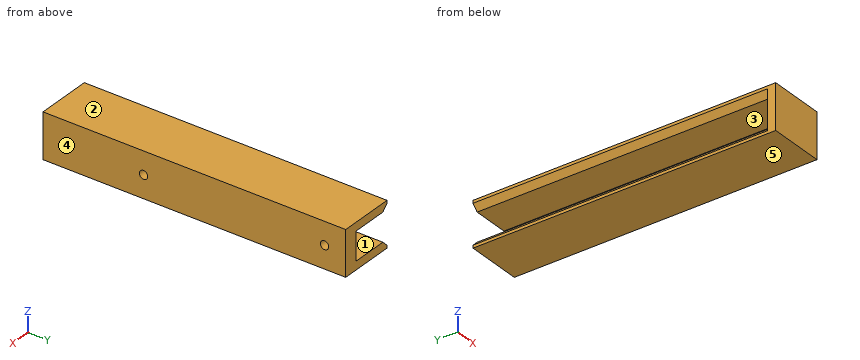
from build123d import *

# Parameters (mm, degrees)
SKETCH_1_W      = 10
SKETCH_1_H      = 105.5
SKETCH_1_R      = 1.6
SKETCH_1_H_2    = 0.1
SKETCH_1_R_2    = 1.5
EXTRUDE_1_DEPTH = 5
EXTRUDE_2_DEPTH = 105.7
CHAMFER_1_SIZE  = 2
EXTRUDE_3_DEPTH = 3


with BuildPart() as part:
    # ｽｹｯﾁ1 → ﾎﾞｽ - 押し出し1 (new body)
    # profile 1 of 5: a face of its own
    with BuildSketch(Plane(origin=(-2.03481113, 0, 0), x_dir=(0, 0, -1), z_dir=(1, 0, 0))):
        with Locations((-131, -7.323272389)):
            Rectangle(SKETCH_1_W, SKETCH_1_H)
        with Locations((-131, -27.073272389)):
            Circle(SKETCH_1_R, mode=Mode.SUBTRACT)
        with Locations((-131, 37.926727611)):
            Circle(SKETCH_1_R, mode=Mode.SUBTRACT)
    # profile 2 of 5: a face of its own
    with BuildSketch(Plane(origin=(-2.03481113, 0, 0), x_dir=(0, 0, -1), z_dir=(1, 0, 0))):
        Polygon((-136, -60.073272389), (-136, 45.426727611), (-136, 45.526727611), (-136.1, 45.526727611), (-136.1, -60.173272389), (-125.9, -60.173272389), (-125.9, 45.526727611), (-126, 45.526727611), (-126, 45.426727611), (-126, -60.073272389), align=None)
    # profile 3 of 5: a face of its own
    with BuildSketch(Plane(origin=(-2.03481113, 0, 0), x_dir=(0, 0, -1), z_dir=(1, 0, 0))):
        with Locations((-131, 45.476727611)):
            Rectangle(SKETCH_1_W, SKETCH_1_H_2)
    # profile 4 of 5: a face of its own
    with BuildSketch(Plane(origin=(-2.03481113, 0, 0), x_dir=(0, 0, -1), z_dir=(1, 0, 0))):
        with Locations((-131, 37.926727611)):
            Circle(SKETCH_1_R)
        with Locations((-131, 37.926727611)):
            Circle(SKETCH_1_R_2, mode=Mode.SUBTRACT)
    # profile 5 of 5: a face of its own
    with BuildSketch(Plane(origin=(-2.03481113, 0, 0), x_dir=(0, 0, -1), z_dir=(1, 0, 0))):
        with Locations((-131, -27.073272389)):
            Circle(SKETCH_1_R)
        with Locations((-131, -27.073272389)):
            Circle(SKETCH_1_R_2, mode=Mode.SUBTRACT)
    extrude(amount=EXTRUDE_1_DEPTH)

    # ｽｹｯﾁ2 → ﾎﾞｽ - 押し出し2 (add)
    with BuildSketch(Plane.XZ.offset(60.173272389)):
        Polygon((2.96518887, 139.1), (-17.03481113, 139.1), (-17.03481113, 136.1), (-2.03481113, 136.1), (2.96518887, 136.1), align=None)
        Polygon((2.96518887, 122.9), (2.96518887, 125.9), (-2.03481113, 125.9), (-17.03481113, 125.9), (-17.03481113, 122.9), align=None)
    extrude(amount=-EXTRUDE_2_DEPTH)

    # 面取り1
    chamfer_1_edges = [part.edges().sort_by_distance(p)[0] for p in [
        (-17.03481113, -7.323272389, 136.1),
        (-17.03481113, -7.323272389, 125.9),
    ]]
    chamfer(chamfer_1_edges, length=CHAMFER_1_SIZE)

    # ｽｹｯﾁ3 → ﾎﾞｽ - 押し出し3 (add)
    with BuildSketch(Plane.XZ.offset(60.173272389)):
        Polygon((-2.03481113, 136.1), (-2.03481113, 125.9), (-15.03481113, 125.9), (-17.03481113, 123.9), (-17.03481113, 122.9), (2.96518887, 122.9), (2.96518887, 139.1), (-17.03481113, 139.1), (-17.03481113, 138.1), (-15.03481113, 136.1), align=None)
        Polygon((-15.03481113, 136.1), (-17.03481113, 138.1), (-17.03481113, 123.9), (-15.03481113, 125.9), (-2.03481113, 125.9), (-2.03481113, 136.1), align=None)
    extrude(amount=EXTRUDE_3_DEPTH)


solid = part.part
Verification items for the finished model (mm, model axes). Face numbers are marked on the shaded views. A direction names the side the tool comes from. Round coordinates to 2 decimals unless told otherwise and drop trailing zeros. Order: outer loops, then holes, each group sorted by start corner. A loop starts at its lowest first (then second) coordinate and runs counter-clockwise, first axis right, second up. Notation, with made-up numbers: (3, 27.25) -> (28, 27.25) arc R21 ccw to (28, 49.25) -> close; hole circle Ø2 at (-21, 67.5). An arc over 180 degrees is marked (long way). Put each result on its own line as item: value.
1) Section check C-C (y = -5.5). Record the cut outline in (x, z), then the cut area to 3 significant figures.
Final values:
outline: (-17.03, 122.9) -> (2.97, 122.9) -> (2.97, 139.1) -> (-17.03, 139.1) -> (-17.03, 138.1) -> (-15.03, 136.1) -> (-2.03, 136.1) -> (-2.03, 125.9) -> (-15.03, 125.9) -> (-17.03, 123.9) -> close
area: 167 mm^2
2) Section check A-A (z = 131). Record the cut outline in (x, y).
Final values:
outline: (-17.03, -63.17) -> (2.97, -63.17) -> (2.97, -28.57) -> (-2.03, -28.57) -> (-2.03, -60.17) -> (-17.03, -60.17) -> close; (-2.03, -25.57) -> (2.97, -25.57) -> (2.97, 36.43) -> (-2.03, 36.43) -> close; (-2.03, 39.43) -> (2.97, 39.43) -> (2.97, 45.53) -> (-2.03, 45.53) -> close
3) Mould release check, pull along Z, two halves, no side actions. Record for the marked faces 3, 4 and 5: +Z half, -Z half, draft (parallel to the pull), parting line (faces both ways), or undercut.
Final values:
face 3: undercut
face 4: draft
face 5: -Z half
4) Section check B-B (x = -8). Record the cut outline in (y, z), then the cut area to 3 significant figures.
Final values:
outline: (-63.17, 122.9) -> (45.53, 122.9) -> (45.53, 125.9) -> (-60.17, 125.9) -> (-60.17, 136.1) -> (45.53, 136.1) -> (45.53, 139.1) -> (-63.17, 139.1) -> close
area: 683 mm^2
5) Depth check by flat-ended pin: pin 1 (3 mm diameter, centred on y = 14, z = 129.5, fed in from -X); pin 2 (2 mm diameter, centred on x = -10, z = 134, fed in from +Y); pin 3 (4 mm diameter, centred on y = -27.07, z = 131, fed in from +X). Enter the tip coordinate at first touch or a pass-through.
Final values:
pin 1: stops at x = -2.03
pin 2: stops at y = -60.17
pin 3: stops at x = 2.97
6) Set-up check for the marked faces 1 and 2: record each of +Z, -Z, +X, -X, +Y, -Y from which the full face is reachable in a straight line by a thin tool's end or side.
Final values:
face 1: -X, +Y
face 2: +Z, +X, -X, +Y, -Y
7) Material ranges on line 1 (Y direction, x = -0.4, z = 131); line 2 (Z direction, x = -8.75, y = -34.5); line 3 (Y direction, x = -8.25, z = 132.75), recorded low to high.
Final values:
line 1: y = -63.17 to -28.57, -25.57 to 36.43, 39.43 to 45.53
line 2: z = 122.9 to 125.9, 136.1 to 139.1
line 3: y = -63.17 to -60.17
